from build123d import *

# Parameters (mm, degrees)
F0_W   = 2.101484
F0_H   = 6
F0_H_2 = 3


with BuildPart() as f1:
    # F0 (on Front) → F1 (revolve)
    with BuildSketch(Plane.XZ):
        with Locations((36.050742, 18.5)):
            Rectangle(F0_W, F0_H)
        Polygon((35, 15.5), (40, 0), (42.101484, 0), (37.101484, 15.5), align=None)
        with Locations((41.050742, -1.5)):
            Rectangle(F0_W, F0_H_2)
    revolve(axis=Axis((0, 0, 7.75), (0, 0, 1)))


solid = f1.part
Geometry check sheet. Reference: the model listing, model coordinates, mm. A direction names the side the tool comes from. Give positions to 0.01 mm unless a question says otherwise; leave off trailing zeros. Order: outer loops, then holes, each group sorted by start corner. A loop starts at its lowest first (then second) coordinate and runs counter-clockwise, first axis right, second up. Notation, with made-up numbers: M 35.25,-33.75 L 50.25,-33.75 A14 ccw 50.25,-23.75 Z; hole C 79.25,64 d4. An arc over 180 degrees is marked long. Use a Markdown table: item, result.
Item 1: Tool access check on faces 4 (the flat face through (22.2, -27.3, 21.5)), 5 (the cylindrical face through (-29.44, -22.58, 18.54)), 6 (the cylindrical face through (-8.67, -39.05, -1.48)). Record the directions out of +Z, -Z, +X, -X, +Y, -Y that give a thin tool (end or side, any length) a straight path to the whole face; none if there is none.
Answers follow:
| item | result |
|---|---|
| face 4 | +Z, +X, -X, +Y, -Y |
| face 5 | +Z |
| face 6 | -Z |
Item 2: Draft check along Y on faces 1 (the cylindrical face through (-28, -21, 19)), 2 (the conical face through (35.62, 11.22, 14.75)), 3 (the flat face through (-37.2, -15.4, -3)). Enter one of: +Y half, -Y half, draft (parallel to the pull), parting line (faces both ways), or undercut.
Answers follow:
| item | result |
|---|---|
| face 1 | undercut |
| face 2 | parting line |
| face 3 | draft |
Item 3: Section check D-D (z = 5.25). Record the cut outline in (x, y), and give its area (3 significant figures).
Answers follow:
| item | result |
|---|---|
| outline | C 0,0 d80.82; hole C 0,0 d76.61 |
| area | 520 mm2 |
Item 4: Section check C-C (z = 19.75). Record the cut outline in (x, y).
Answers follow:
| item | result |
|---|---|
| outline | C 0,0 d74.2; hole C 0,0 d70 |
Item 5: Depth check by flat-ended pin: P1, Ø3, axis at y = 0, z = 18.5, coming from the +X side; P2, Ø12, axis at x = -16, z = 11, coming from the +Y side; P3, Ø1, axis at x = -31.5, z = 0, coming from the +Y side. Enter the tip coordinate at first touch or a pass-through.
Answers follow:
| item | result |
|---|---|
| P1 | stops at x = 37.1 |
| P2 | stops at y = 38.15 |
| P3 | stops at y = 28.49 |
Item 6: Section check A-A (y = 0). Record the cut outline in (x, z).
Answers follow:
| item | result |
|---|---|
| outline | M -42.1,-3 L -40,-3 L -40,0 L -35,15.5 L -35,21.5 L -37.1,21.5 L -37.1,15.5 L -42.1,0 Z; M 35,15.5 L 40,0 L 40,-3 L 42.1,-3 L 42.1,0 L 37.1,15.5 L 37.1,21.5 L 35,21.5 Z |
Item 7: Material ranges on line 1 along Y through (x, z) = (0, 19.8); line 2 along Y through (x, z) = (-8, 1); line 3 along X through (y, z) = (-10, 19), recorded low to high.
Answers follow:
| item | result |
|---|---|
| line 1 | y = -37.1 to -35, 35 to 37.1 |
| line 2 | y = -41.01 to -38.86, 38.86 to 41.01 |
| line 3 | x = -35.73 to -33.54, 33.54 to 35.73 |
